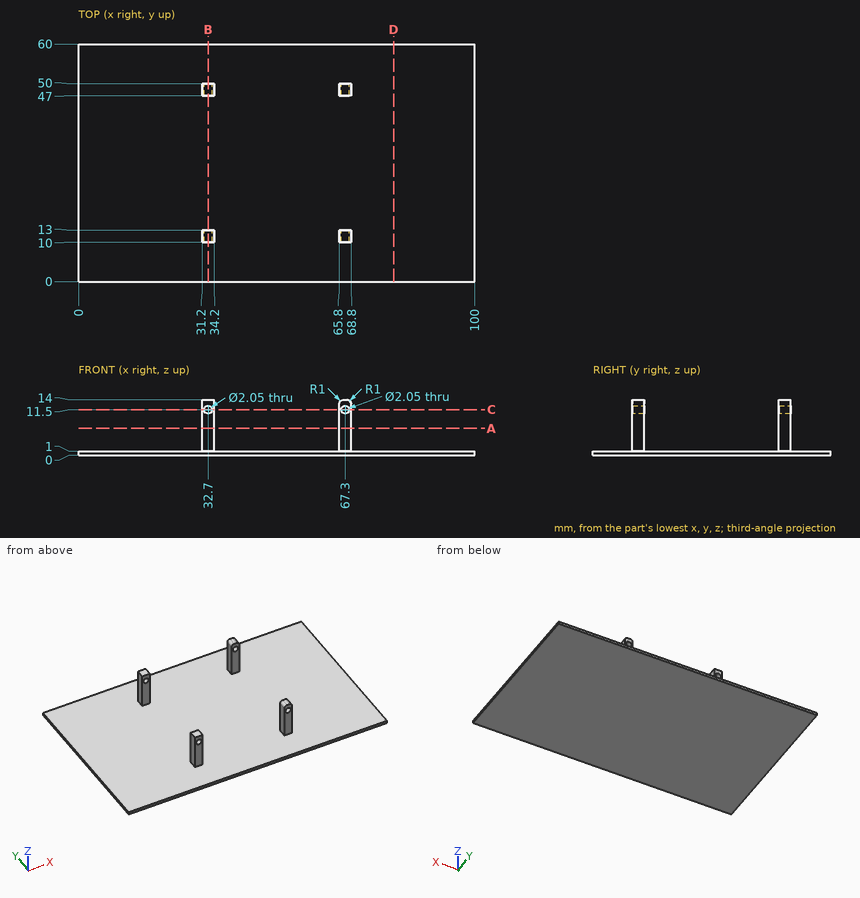
Design review of the part shown in the three views and the two pictorial views. Dimensions are in mm from the part's minimum x, y and z. Round coordinates to 2 decimals unless told otherwise and drop trailing zeros. Write each loop counter-clockwise with the first axis right and the second up, starting at its lowest first coordinate (ties: lowest second). Pieces come first, ordered by that corner, then holes. Notation, with made-up numbers: (-20.5, -36) - (5.5, -36) arc R14 cw to (5.5, -12) - close; hole circle Ø9 at (24, 51.25). An arc over 180 degrees is marked (long way). Return JSON: item names as keys, results as strings. Group by question number.
Item 1: We need section B-B on x = 32.7. Write out the cut boundary in (y, z) (3 decimals).
Item 2: We need section D-D on x = 79.5. Write out the cut boundary in (y, z), and give its area (3 significant figures).
Item 3: We need section A-A on z = 6.75. Write out the cut boundary in (x, y).
Item 4: For probe 1 along X at (y, z) = (48.4, 11.5) (3 decimals); probe 2 along Z at (x, y) = (32.7, 48) (3 decimals); probe 3 along X at (y, z) = (49, 1.5), list the stretches that pass through material, from the lowest coordinate up. Write a range as [from, to].
Item 5: We need section C-C on z = 11.5. Give the number of separate pieces and of enclosed holes in the cut face, and give its area (3 significant figures).
Item 6: Insertion check: P1, Ø3, axis at y = 7, z = 10, coming from the -X side; P2, Ø0.9, axis at y = 12, z = 8.5, coming from the -X side; P3, Ø1.5, axis at y = 11, z = 4.5, coming from the +X side; P4, Ø1.5, axis at x = 67, z = 6.5, coming from the -Y side. Each pin has a flat end and moves straight along its axis. Give the tip position at first contact, or say it passes through.
Model answer:
{
 "1": {"outline": "(0, 0) - (60, 0) - (60, 1) - (50, 1) - (50, 10.475) - (47, 10.475) - (47, 1) - (13, 1) - (13, 10.475) - (10, 10.475) - (10, 1) - (0, 1) - close; (10, 12.525) - (13, 12.525) - (13, 14) - (10, 14) - close; (47, 12.525) - (50, 12.525) - (50, 14) - (47, 14) - close"},
 "2": {"outline": "(0, 0) - (60, 0) - (60, 1) - (0, 1) - close", "area": "60.0 mm²"},
 "3": {"outline": "(31.2, 10) - (34.2, 10) - (34.2, 13) - (31.2, 13) - close; (31.2, 47) - (34.2, 47) - (34.2, 50) - (31.2, 50) - close; (65.8, 10) - (68.8, 10) - (68.8, 13) - (65.8, 13) - close; (65.8, 47) - (68.8, 47) - (68.8, 50) - (65.8, 50) - close"},
 "4": {"probe 1": "x = [31.2, 31.675], [33.725, 34.2], [65.8, 66.275], [68.325, 68.8]", "probe 2": "z = [0, 10.475], [12.525, 14]", "probe 3": "x = [31.2, 34.2], [65.8, 68.8]"},
 "5": {"separate pieces": "8", "enclosed holes": "0", "area": "11.4 mm²"},
 "6": {"P1": "passes through", "P2": "stops at x = 31.2", "P3": "stops at x = 68.8", "P4": "stops at y = 10"}
}
